Source: CAD feature listing. Evaluate the final solid. Frame: model axes, mm. Round coordinates to 2 decimals unless told otherwise and drop trailing zeros. Loops run counter-clockwise (first coordinate to the right, second up) from the corner with the lowest first, then second, coordinate; pieces in that order, holes last.
(1) First-contact query: pin 1 Ø1.5 at (x, z) = (17, 499) entering from +Y; pin 2 Ø4 at (x, z) = (0, 421) entering from +Y; pin 3 Ø8 at (x, z) = (15, 1001) entering from +Y. Flat tips, straight axial feed; report the tip coordinate or a pass-through.
(2) Material intervals for probe 1 along X at (y, z) = (12.25, 793) (3 decimals); probe 2 along Y at (x, z) = (-1, 428.5) (3 decimals); probe 3 along X at (y, z) = (1.3, 421) (3 decimals), sorted ascending.
(3) Section A-A, the plane y = 12. Return the cut outline in (x, z) (3 decimals), plus the area to 3 significant figures.
(4) Section B-B, the plane z = 512. Return the cut outline in (x, y) (1 decimal).
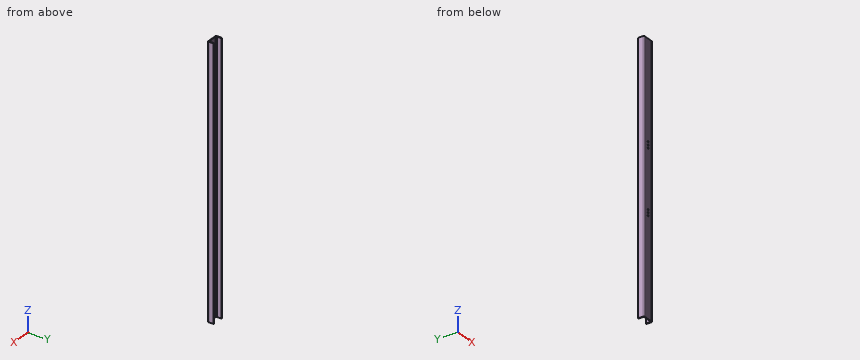
```python
from build123d import *

# Parameters (mm, degrees)
BOSS_EXTRUDE1_DEPTH         = 1143
FILLET1_R                   = 4.7625
FILLET2_R                   = 4.7625
F_1_4_0_25_DIAMETER_HOLE1_D = 6.35


with BuildPart() as part:
    # Sketch1 → Boss-Extrude1 (new body)
    with BuildSketch(Plane.XY):
        Polygon((-25.4, 25.4), (-25.4, 0), (25.4, 0), (25.4, 25.4), (22.225, 25.4), (22.225, 3.175), (-22.225, 3.175), (-22.225, 25.4), align=None)
    extrude(amount=BOSS_EXTRUDE1_DEPTH)

    # Fillet1
    fillet1_edges = [part.edges().sort_by_distance(p)[0] for p in [
        (-22.225, 3.175, 571.5),
        (22.225, 3.175, 571.5),
    ]]
    fillet(fillet1_edges, radius=FILLET1_R)

    # Fillet2
    fillet2_edges = [part.edges().sort_by_distance(p)[0] for p in [
        (25.4, 0, 571.5),
        (-25.4, 0, 571.5),
    ]]
    fillet(fillet2_edges, radius=FILLET2_R)

    # 1/4 (0.25) Diameter Hole1 (through all)
    with Locations(Plane(origin=(0, 3.175, 0), x_dir=(1, 0, 0), z_dir=(0, 1, 0))):
        with Locations((0, -722), (0, -709.3), (0, -696.6), (0, -446.4), (0, -433.7), (0, -421)):
            Hole(F_1_4_0_25_DIAMETER_HOLE1_D / 2)


solid = part.part
```
Output values:
1. pin 1: stops at y = 3.18
1. pin 2: passes through
1. pin 3: stops at y = 3.43
2. probe 1: x = -25.4 to -22.225, 22.225 to 25.4
2. probe 2: y = 0 to 3.175
2. probe 3: x = -23.907 to -3.175, 3.175 to 23.907
3. outline: (-25.4, 0) - (-22.225, 0) - (-22.225, 1143) - (-25.4, 1143) - close; (22.225, 0) - (25.4, 0) - (25.4, 1143) - (22.225, 1143) - close
3. area: 7,260 mm2
4. outline: (-25.4, 4.8) arc R4.8 ccw to (-20.6, 0) - (20.6, 0) arc R4.8 ccw to (25.4, 4.8) - (25.4, 25.4) - (22.2, 25.4) - (22.2, 7.9) arc R4.8 cw to (17.5, 3.2) - (-17.5, 3.2) arc R4.8 cw to (-22.2, 7.9) - (-22.2, 25.4) - (-25.4, 25.4) - close
